Answer from the drawing. Dimensions are ordinates in mm from the lowest x, y and z of the part. Round coordinates to 2 decimals unless told otherwise and drop trailing zeros. Loops run counter-clockwise (first coordinate to the right, second up) from the corner with the lowest first, then second, coordinate; pieces in that order, holes last. Notation, with made-up numbers: (9.25, 66) - (67.25, 66) arc R26 ccw to (67.25, 84) - close; hole circle Ø10 at (9.25, 5). An arc over 180 degrees is marked (long way). Answer as CSV lines item,"result". Start each with the question number.
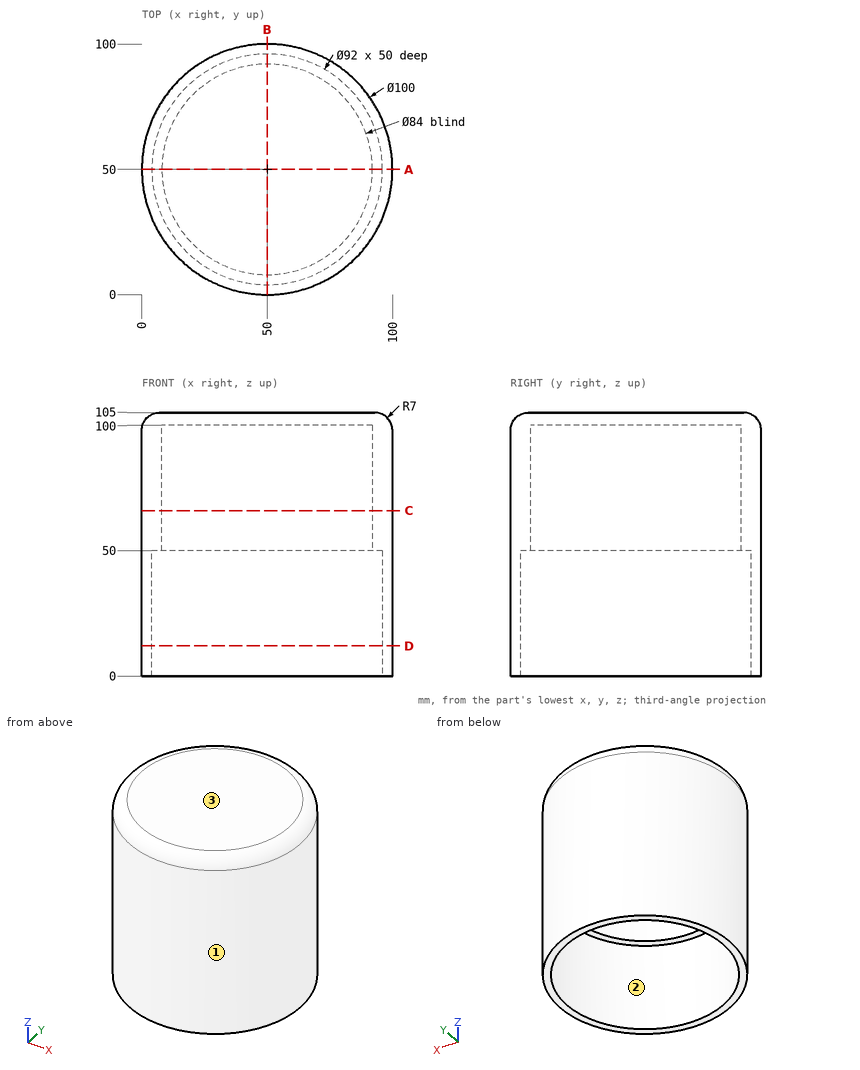
Item 1: Section D-D, the plane z = 12 is taken. Give the vertices of the cut face in (x, y).
Item 2: Find the intervals of material crossed by L1, parallel to Y at x = 50, z = 28.5; L2, parallel to Y at x = 50, z = 89; L3, parallel to X at y = 80, z = 88, in increasing order.
Item 3: Section C-C, the plane z = 66 is taken. Give the vertices of the cut face in (x, y), and give its area (3 significant figures).
Item 4: Flat-ended cylindrical pins translate along their axes: pin 1 Ø10 at (x, z) = (17, 72.5) entering from +Y; pin 2 Ø1 at (x, y) = (28.5, 72) entering from -Z; pin 3 Ø10 at (x, z) = (21.5, 86.5) entering from -Y; pin 4 Ø10 at (y, z) = (53, 83) entering from +X. Find the tip coordinate at first contact, or state that the pin passes through.
Item 5: Section A-A, the plane y = 50 is taken. Give the vertices of the cut face in (x, z), and give its area (3 significant figures).
Item 6: Determine the mould class of the marked faces 1, 2 and 3 for opening direction Y: pulls with the +Y half, pulls with the -Y half, needs draft (parallel to the pull), parting line crosses it, or undercut.
Answer:
1,outline,"circle Ø100 at (50, 50); hole circle Ø92 at (50, 50)"
2,L1,"y = 0 to 4, 96 to 100"
2,L2,"y = 0 to 8, 92 to 100"
2,L3,"x = 10 to 20.61, 79.39 to 90"
3,outline,"circle Ø100 at (50, 50); hole circle Ø84 at (50, 50)"
3,area,"2,310 mm²"
4,pin 1,"stops at y = 91.42"
4,pin 2,"stops at z = 100"
4,pin 3,"stops at y = 5.87"
4,pin 4,"stops at x = 100"
5,outline,"(0, 0) - (4, 0) - (4, 50) - (8, 50) - (8, 100) - (92, 100) - (92, 50) - (96, 50) - (96, 0) - (100, 0) - (100, 98) arc R7 ccw to (93, 105) - (7, 105) arc R7 ccw to (0, 98) - close"
5,area,"1,680 mm²"
6,face 1,"parting line crosses it"
6,face 2,"undercut"
6,face 3,"needs draft"
